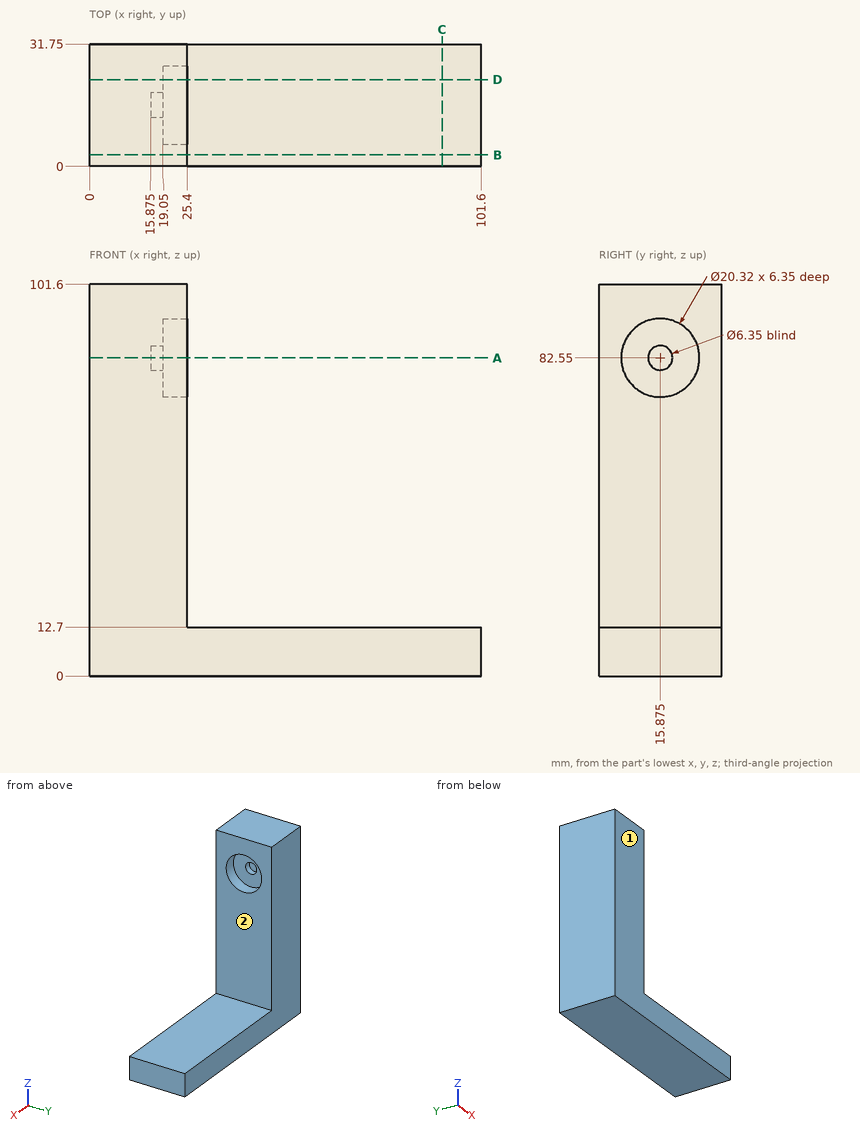
Here's the drawing with two shaded views (mm, measured from the low corner). I have some questions. A direction names the side the tool comes from. Give positions to 0.01 mm unless a question says otherwise; leave off trailing zeros. Write each loop counter-clockwise with the first axis right and the second up, starting at its lowest first coordinate (ties: lowest second). Pieces come first, ordered by that corner, then holes. Notation, with made-up numbers: (-21, -9.75) - (15, -9.75) arc R16 cw to (15, 18.25) - close; hole circle Ø7 at (71, 89.25). An arc over 180 degrees is marked (long way). Write item = value, one per line. Start each with the question number.
1. Imagine slicing it at C-C (x = 91.5). Please give me the cut outline in (y, z), and give its area (3 significant figures).
2. For pin 1 (12 mm diameter, centred on x = 44, y = 14.5, fed in from +Z); pin 2 (10 mm diameter, centred on y = 12.5, z = 82.5, fed in from +X); pin 3 (12 mm diameter, centred on y = 11, z = 78.5, fed in from +X), each with a flat end and sliding along its axis, tell me the tip position at first contact or that it passes through.
3. On a 3-axis mill with a long thin cutter (end or side, diameter ignored), from which of +Z, -Z, +X, -X, +Y, -Y can I reach the whole of each face in a straight line? I mean the marked faces 1 and 2. Say none if no direction works.
4. Please list where these lines run through material, in increasing order: line 1 (Y direction, x = 20, z = 82); line 2 (X direction, y = 2, z = 71); line 3 (Z direction, x = 77.5, y = 23.5).
5. Imagine slicing it at D-D (y = 22.5). Please give me the cut outline in (x, z).
6. Imagine slicing it at B-B (y = 3). Please give me the cut outline in (x, z).
7. Imagine slicing it at A-A (z = 82.55). Please give me the cut outline in (x, y) (3 decimals).
Worked answers:
q1.outline = (0, 0) - (31.75, 0) - (31.75, 12.7) - (0, 12.7) - close
q1.area = 403 mm2
q2.pin_1 = 12.7
q2.pin_2 = 19.05
q2.pin_3 = 25.4
q3.face_1 = +Z, -Z, +X, -X, -Y
q3.face_2 = +Z, +X, +Y, -Y
q4.line_1 = 0 to 5.73, 26.02 to 31.75
q4.line_2 = 0 to 25.4
q4.line_3 = 0 to 12.7
q5.outline = (0, 0) - (101.6, 0) - (101.6, 12.7) - (25.4, 12.7) - (25.4, 74.85) - (19.05, 74.85) - (19.05, 90.25) - (25.4, 90.25) - (25.4, 101.6) - (0, 101.6) - close
q6.outline = (0, 0) - (101.6, 0) - (101.6, 12.7) - (25.4, 12.7) - (25.4, 101.6) - (0, 101.6) - close
q7.outline = (0, 0) - (25.4, 0) - (25.4, 5.715) - (19.05, 5.715) - (19.05, 12.7) - (15.875, 12.7) - (15.875, 19.05) - (19.05, 19.05) - (19.05, 26.035) - (25.4, 26.035) - (25.4, 31.75) - (0, 31.75) - close
